Geometry: final body of the model. Coordinates: model frame, mm. Give positions to 0.01 mm unless a question says otherwise; leave off trailing zeros. Order: outer loops, then holes, each group sorted by start corner. A loop starts at its lowest first (then second) coordinate and runs counter-clockwise, first axis right, second up. Notation, with made-up numbers: M -14,-36 L 22,-36 A23 ccw 22,0 Z; hole C 5,12.5 d6. An arc over 180 degrees is marked long. One line per item, written item: value. Start each with the question number.
```python
from build123d import *

# Parameters (mm, degrees)
SKETCH1_R           = 1.896979128
SKETCH1_R_2         = 1.786033574
SKETCH1_R_3         = 2
SKETCH1_R_4         = 7
BOSS_EXTRUDE1_DEPTH = 1.5875
SKETCH4_W           = 66.272407177
SKETCH4_H           = 27.800260981
CUT_EXTRUDE2_DEPTH  = 20
FILLET3_R           = 10
FILLET4_R           = 10
BOSS_EXTRUDE3_START = -1.5875
BOSS_EXTRUDE3_DEPTH = 1.5875
SKETCH7_R           = 7
CUT_EXTRUDE3_DEPTH  = 1.5875


with BuildPart() as part:
    # Sketch1 → Boss-Extrude1 (new body)
    with BuildSketch(Plane(origin=(0, 0, 0), x_dir=(1, 0, 0), z_dir=(0, 1, 0))):
        with BuildLine():
            Line((42.32729629, 228.6), (10.454309325, 228.6))
            Line((10.454309325, 228.6), (0, 135.362739137))
            Line((0, 135.362739137), (0, 0))
            Line((0, 0), (24.327009544, 0))
            Line((24.327009544, 0), (50.8, 0))
            Line((50.8, 0), (50.8, 64.87909603))
            Line((50.8, 64.87909603), (50.8, 87.423477361))
            Line((50.8, 87.423477361), (50.8, 98.200996728))
            ThreePointArc((50.8, 98.200996728), (50.4, 101.000996728), (50.8, 103.800996728))
            Line((50.8, 103.800996728), (50.8, 104.488200565))
            Line((50.8, 104.488200565), (50.8, 120.619222808))
            Line((50.8, 120.619222808), (50.8, 135.362739137))
            Line((50.8, 135.362739137), (42.32729629, 228.6))
        make_face()
        with Locations(Location((17.418441927, 23.081717093, 0), (0, 0, 270))):
            Circle(SKETCH1_R, mode=Mode.SUBTRACT)
        with Locations(Location((17.127384385, 39.079069546, 0), (0, 0, 270))):
            Circle(SKETCH1_R_2, mode=Mode.SUBTRACT)
        with Locations(Location((33.41579438, 23.372774635, 0), (0, 0, 270))):
            Circle(SKETCH1_R_3, mode=Mode.SUBTRACT)
        with Locations(Location((33.124736838, 39.370127088, 0), (0, 0, 270))):
            Circle(SKETCH1_R_3, mode=Mode.SUBTRACT)
        with BuildLine():
            Line((34.925740903, 92.78493524), (9.492033273, 92.78493524))
            ThreePointArc((9.492033273, 92.78493524), (6.992033273, 95.28493524), (9.492033273, 97.78493524))
            Line((9.492033273, 97.78493524), (34.925740903, 97.78493524))
            ThreePointArc((34.925740903, 97.78493524), (36.693507856, 97.052702193), (37.425740903, 95.28493524))
            ThreePointArc((37.425740903, 95.28493524), (36.693507856, 93.517168287), (34.925740903, 92.78493524))
        make_face(mode=Mode.SUBTRACT)
        with BuildLine():
            Line((34.925740903, 105.90993524), (9.492033273, 105.90993524))
            ThreePointArc((9.492033273, 105.90993524), (6.492033273, 108.90993524), (9.492033273, 111.90993524))
            Line((9.492033273, 111.90993524), (34.925740903, 111.90993524))
            ThreePointArc((34.925740903, 111.90993524), (37.047061246, 111.031255584), (37.925740903, 108.90993524))
            ThreePointArc((37.925740903, 108.90993524), (37.047061246, 106.788614896), (34.925740903, 105.90993524))
        make_face(mode=Mode.SUBTRACT)
        with BuildLine():
            Line((35.509675341, 119.784935244), (9.492033273, 119.784935244))
            ThreePointArc((9.492033273, 119.784935244), (7.026609419, 122.250359097), (9.492033273, 124.71578295))
            Line((9.492033273, 124.71578295), (35.509675341, 124.71578295))
            ThreePointArc((35.509675341, 124.71578295), (37.252993266, 123.993677022), (37.975099194, 122.250359097))
            ThreePointArc((37.975099194, 122.250359097), (37.252993266, 120.507041172), (35.509675341, 119.784935244))
        make_face(mode=Mode.SUBTRACT)
        with Locations(Location((29.504213454, 189.557234372, 0), (0, 0, 270))):
            Circle(SKETCH1_R_4, mode=Mode.SUBTRACT)
    extrude(amount=BOSS_EXTRUDE1_DEPTH)

    # Sketch4 → Cut-Extrude2 (cut)
    with BuildSketch(Plane(origin=(0, 0, -228.6), x_dir=(-1, 0, 0), z_dir=(0, 0, -1))):
        with Locations((-28.174690156, -1.980940155)):
            Rectangle(SKETCH4_W, SKETCH4_H)
    extrude(amount=-CUT_EXTRUDE2_DEPTH, mode=Mode.SUBTRACT)

    # Fillet3
    fillet3_edges = [part.edges().sort_by_distance(p)[0] for p in [
        (44.144746445, 0.79375, -208.6),
    ]]
    fillet(fillet3_edges, radius=FILLET3_R)

    # Fillet4
    fillet4_edges = [part.edges().sort_by_distance(p)[0] for p in [
        (50.8, 0.79375, 0),
        (0, 0.79375, 0),
        (8.211791854, 0.79375, -208.6),
    ]]
    fillet(fillet4_edges, radius=FILLET4_R)

    # Sketch6 → Boss-Extrude3 (add)
    with BuildSketch(Plane(origin=(0, 1.5875, 0), x_dir=(1, 0, 0), z_dir=(0, 1, 0)).offset(BOSS_EXTRUDE3_START)):
        with BuildLine():
            Line((50.8, 135.362739137), (50.8, 103.800996728))
            ThreePointArc((50.8, 103.800996728), (50.4, 101.000996728), (50.8, 98.200996728))
            Line((50.8, 98.200996728), (50.8, 61.124243317))
            Line((50.8, 61.124243317), (69.258211507, 96.360728536))
            ThreePointArc((69.258211507, 96.360728536), (70.393157133, 101.370875786), (68.890940865, 106.283413148))
            Line((68.890940865, 106.283413148), (50.8, 135.362739137))
        make_face()
    extrude(amount=BOSS_EXTRUDE3_DEPTH)

    # Sketch7 → Cut-Extrude3 (cut)
    with BuildSketch(Plane(origin=(0, 1.5875, 0), x_dir=(1, 0, 0), z_dir=(0, 1, 0))):
        with Locations(Location((60.4, 101.000996728, 0), (0, 0, 270))):
            Circle(SKETCH7_R)
    extrude(amount=-CUT_EXTRUDE3_DEPTH, mode=Mode.SUBTRACT)


solid = part.part
```
Q1. Section query A-A on x = 60.4. Return loops of the section in (y, z), and give its area (3 significant figures).
Q2. Contact query for flat-ended pins moving along their axis: pin 1 (0.5 mm diameter, centred on x = 16.5, y = 1, fed in from -Z); pin 2 (11 mm diameter, centred on x = 60.4, z = -101, fed in from -Y); pin 3 (0.5 mm diameter, centred on y = 0.5, z = -46, fed in from +X). Output: stop coordinate, or through.
Q3. Section query C-C on z = -56.5. Return loops of the section in (x, y).
Q4. Ray query, line 1 along Z through (x, y) = (22, 0.45); line 2 along X through (y, z) = (1.2, -96.5); line 3 along Z through (x, y) = (8, 1.05). Return the intervals inside material, ascending. Write a range as [from, to].
Q5. Section query D-D on z = -170. Return loops of the section in (x, y).
Q6. Section query B-B on y = 1.15. Give the number of separate pieces and of enclosed holes in the cut face, and give its area (3 significant figures).
Q7. Mould query, pull axis X, two halves, no side actions, for faces 1 (the face through (57.719, 0.805, -94.535)), 2 (the face through (59.97, 0.78, -120.62)), 3 (the face through (43, 0, -106)). Classes: +X half, -X half, draft (parallel to the pull), parting line (faces both ways), or undercut.
Results below:
1. outline: M 0,-119.93 L 1.59,-119.93 L 1.59,-108 L 0,-108 Z; M 0,-94 L 1.59,-94 L 1.59,-79.45 L 0,-79.45 Z
1. area: 42.0 mm2
2. pin 1: z = -208.59
2. pin 2: through
2. pin 3: x = 50.8
3. outline: M 0,0 L 50.8,0 L 50.8,1.59 L 0,1.59 Z
4. line 1: [-208.6, -124.72], [-119.78, -111.91], [-105.91, -97.78], [-92.78, 0]
4. line 2: [0, 7.31], [37.11, 55.04], [65.76, 69.33]
4. line 3: [-202.63, -124.21], [-120.29, -111.51], [-106.31, -97.29], [-93.28, -0.2]
5. outline: M 3.88,0 L 47.65,0 L 47.65,1.59 L 3.88,1.59 Z
6. separate pieces: 1
6. enclosed holes: 9
6. area: 9,920 mm2
7. face 1: undercut
7. face 2: +X half
7. face 3: draft
